The listing builds one solid part. Answer for the finished solid, in the listing's coordinates (mm). Coordinates: 2 decimals unless noted, no trailing zeros. Loops run counter-clockwise (first coordinate to the right, second up) from the corner with the lowest first, then second, coordinate; pieces in that order, holes last. Notation, with made-up numbers: (4.5, -5.5) - (58.5, -5.5) arc R21 cw to (58.5, 1.5) - close; hole circle Ø3 at (-11, 5). An arc over 180 degrees is marked (long way). Put each result on its own line as item: value.
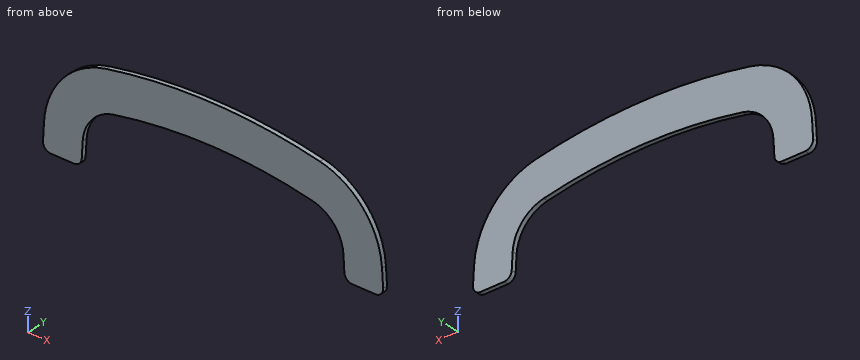
```python
from build123d import *

# Parameters (mm, degrees)
F1_DEPTH = 18
F2_R     = 300
F4_DEPTH = 18.0010001
F5_R     = 30


# Not quite as in the source:
# - a feature names something its author has since deleted; it is built from what else it names


with BuildPart() as f1:
    # F0 (on Front) → F1 (new body)
    with BuildSketch(Plane.XZ):
        with BuildLine():
            Line((-685, 200), (-685, 0))
            Line((-685, 0), (685, 0))
            Line((685, 0), (685, 200))
            ThreePointArc((685, 200), (673.7460477003, 800.4217267888), (640, 1400))
            ThreePointArc((640, 1400), (0, 1500), (-640, 1400))
            ThreePointArc((-640, 1400), (-673.7460477003, 800.4217267888), (-685, 200))
        make_face()
    extrude(amount=F1_DEPTH)

    # F2
    f2_edges = [f1.edges().sort_by_distance(p)[0] for p in [
        (-640, -9, 1400),
        (640, -9, 1400),
    ]]
    fillet(f2_edges, radius=F2_R)

    # F3 (on face) → F4 (cut, through all)
    with BuildSketch(Plane.XZ.offset(18)):
        with BuildLine():
            ThreePointArc((-385.0351790184, 1311.5685143294), (-468.492433607, 1263.0523750474), (-505.1041546871, 1173.7298639214))
            ThreePointArc((-505.1041546871, 1173.7298639214), (-507.8289943623, 1128.3346974136), (-510.4237596585, 1082.9319102019))
            Line((-510.4237596585, 1082.9319102019), (-660.6541901542, 1082.9319102019))
            ThreePointArc((-660.6541901542, 1082.9319102019), (-678.9123910716, 641.6337499869), (-685, 200))
            Line((-685, 200), (-685, 0))
            Line((-685, 0), (685, 0))
            Line((685, 0), (685, 200))
            ThreePointArc((685, 200), (678.9123910716, 641.6337499869), (660.6541901542, 1082.9319102019))
            Line((660.6541901542, 1082.9319102019), (510.4237596585, 1082.9319102019))
            ThreePointArc((510.4237596585, 1082.9319102019), (507.8289943623, 1128.3346974136), (505.1041546871, 1173.7298639214))
            ThreePointArc((505.1041546871, 1173.7298639214), (468.492433607, 1263.0523750474), (385.0351790184, 1311.5685143294))
            ThreePointArc((385.0351790184, 1311.5685143294), (0, 1350), (-385.0351790184, 1311.5685143294))
        make_face()
    extrude(amount=-F4_DEPTH, mode=Mode.SUBTRACT)

    # F5
    f5_edges = [f1.edges().sort_by_distance(p)[0] for p in [
        (-510.42376, -9, 1082.93191),
        (510.42376, -9, 1082.93191),
        (-660.65419, -9, 1082.93191),
        (660.65419, -9, 1082.93191),
    ]]
    fillet(f5_edges, radius=F5_R)


solid = f1.part
```
1) Each of these flat-tipped pins is pushed along its axis until it touches: pin 1 (1 mm diameter, centred on x = -413.5, y = -7.5, fed in from +Z); pin 2 (2 mm diameter, centred on y = -14, z = 1294, fed in from -X); pin 3 (1.5 mm diameter, centred on x = 305, y = -6, fed in from -Z); pin 4 (4 mm diameter, centred on x = 486, z = 1329.5, fed in from +Y). Where does it stop, or does it pass through?
Found:
pin 1: stops at z = 1458.95
pin 2: stops at x = -626.49
pin 3: stops at z = 1325.86
pin 4: stops at y = 0
2) The part is cut by section A-A (x = 339). Give the vertices of the cut face in (y, z).
Found:
outline: (-18, 1320.28) - (0, 1320.28) - (0, 1472.43) - (-18, 1472.43) - close
3) The part is cut by section B-B (x = -368.5). Give the vertices of the cut face in (y, z).
Found:
outline: (-18, 1314.83) - (0, 1314.83) - (0, 1467.38) - (-18, 1467.38) - close
4) Straight lines are drawn through the part: L1, parallel to X at y = -13.5, z = 1262.5; L2, parallel to X at y = -10.5, z = 1265; L3, parallel to Z at x = -570, y = -1.5. For each, find the intervals that lie inside material, in ascending order. Write a range as [from, to].
Found:
L1: x = [-638.94, -468.97], [468.97, 638.94]
L2: x = [-638.06, -466.77], [466.77, 638.06]
L3: z = [1082.93, 1374.15]
